Autodesk Inventor part; units mm, degrees
ref_plane "YZ Plane" through (0, 0, 0) normal (1, 0, 0) x (0, 1, 0)
ref_plane "XZ Plane" through (0, 0, 0) normal (0, 1, 0) x (-1, 0, 0)
ref_plane "XY Plane" through (0, 0, 0) normal (0, 0, 1) x (1, 0, 0)
sketch "Sketch1" plane through (0, 0, 0) normal (0, 1, 0) x (-1, 0, 0)
  circle A0 centre (0, 0) radius 50
  circle A1 centre (0, 0) radius 69.85
  dimension "d0" = 139.7
  dimension "d1" = 100
extrude "Extrusion1" add sketch "Sketch1" along normal blind 12.7
sketch "Sketch2" plane through (0, 12.7, 0) normal (0, 1, 0) x (1, 0, 0)
  circle A0 centre (0, 0) radius 69.85
  line L0 (-69.85, 0) -> (-60.325, 0)
  point P0 (-30.1625, 52.243)
  point P1 (30.1625, 52.243)
  point P2 (60.325, 0)
  point P3 (30.1625, -52.243)
  point P4 (-30.1625, -52.243)
  dimension "d4" = 9.525
  dimension "d7" = 360
hole "Hole1" at (-60.325, 12.7, 0) at (-30.1625, 12.7, -52.243) at (30.1625, 12.7, -52.243) at (60.325, 12.7, 0) at (30.1625, 12.7, 52.243) at (-30.1625, 12.7, 52.243) direction (0, -1, 0) diameter 6.5278 end through all
properties part number "BearingRing"
CAD build for the part. Positions are in the model's coordinates, mm. Round coordinates to 2 decimals unless told otherwise and drop trailing zeros. Order: outer loops, then holes, each group sorted by start corner. A loop starts at its lowest first (then second) coordinate and runs counter-clockwise, first axis right, second up. Notation, with made-up numbers: (2.25, 87.5) - (54.25, 87.5) arc R17 ccw to (54.25, 108.5) - close; hole circle Ø3 at (7.25, 70). An arc over 180 degrees is marked (long way). Answer in a Markdown table with one row per item. Add a question column.
(1) Band-saw the part on A-A on x = 0. List the corners of the cut face in (y, z).
(2) Band-saw the part on C-C on y = 3. Count the separate pieces of the cut face and the enclosed holes in it, and give its area (3 significant figures).
(3) Drop flat-ended pins along their axis: pin 1 Ø4 at (x, y) = (40.5, 3) entering from -Z; pin 2 Ø10.5 at (x, z) = (-30.16, 52.24) entering from -Y; pin 3 Ø1.5 at (y, z) = (7, -32) entering from -X; pin 4 Ø1 at (y, z) = (7.5, -8.5) entering from -X. Give the stop position or say it passes through.
(4) Band-saw the part on D-D on z = -29. List the corners of the cut face in (x, y).
(5) Mould opens along Z. For faces 1 (the face through (-46, 12.7, 21)), 2 (the face through (55.431, 6.261, 42.503)), 3 (the face through (-47.69, 6.26, -15.02)) say: +Z half, -Z half, draft (parallel to the pull), parting line (faces both ways), or undercut.
(6) Band-saw the part on B-B on z = 0. List the corners of the cut face in (x, y), and give its area (3 significant figures).
(7) Probe L1, parallel to X at y = 2.75, z = 3; L2, parallel to Z at x = 1.5, y = 4.75; L3, parallel to Z at x = -31.5, y = 11.5. List the from-to ranges inside material, lowest first. Write a range as [from, to].
Data:
| question | item | result |
|---|---|---|
| 1 | outline | (0, -69.85) - (12.7, -69.85) - (12.7, -50) - (0, -50) - close; (0, 50) - (12.7, 50) - (12.7, 69.85) - (0, 69.85) - close |
| 2 | separate pieces | 1 |
| 2 | enclosed holes | 7 |
| 2 | area | 7,270 mm^2 |
| 3 | pin 1 | stops at z = -58.28 |
| 3 | pin 2 | stops at y = 0 |
| 3 | pin 3 | stops at x = -62.47 |
| 3 | pin 4 | stops at x = -69.39 |
| 4 | outline | (-63.55, 0) - (-40.73, 0) - (-40.73, 12.7) - (-63.55, 12.7) - close; (40.73, 0) - (63.55, 0) - (63.55, 12.7) - (40.73, 12.7) - close |
| 5 | face 1 | draft |
| 5 | face 2 | parting line |
| 5 | face 3 | undercut |
| 6 | outline | (-69.85, 0) - (-63.59, 0) - (-63.59, 12.7) - (-69.85, 12.7) - close; (-57.06, 0) - (-50, 0) - (-50, 12.7) - (-57.06, 12.7) - close; (50, 0) - (57.06, 0) - (57.06, 12.7) - (50, 12.7) - close; (63.59, 0) - (69.85, 0) - (69.85, 12.7) - (63.59, 12.7) - close |
| 6 | area | 338 mm^2 |
| 7 | L1 | x = [-69.79, -61.61], [-59.04, -49.91], [49.91, 59.04], [61.61, 69.79] |
| 7 | L2 | z = [-69.83, -49.98], [49.98, 69.83] |
| 7 | L3 | z = [-62.34, -55.22], [-49.27, -38.83], [38.83, 49.27], [55.22, 62.34] |
